Autodesk Inventor part; units mm, degrees
ref_plane "YZ Plane" through (0, 0, 0) normal (1, 0, 0) x (0, 1, 0)
ref_plane "XZ Plane" through (0, 0, 0) normal (0, 1, 0) x (-1, 0, 0)
ref_plane "XY Plane" through (0, 0, 0) normal (0, 0, 1) x (1, 0, 0)
sketch "Esboço1" plane through (0, 0, 0) normal (0, 0, 1) x (1, 0, 0)
  line L0 (0, 0) -> (40, 0)
  line L1 (40, 0) -> (40, 40)
  line L2 (40, 40) -> (0, 40)
  line L3 (0, 40) -> (0, 0)
  dimension "d0" = 40
  dimension "d1" = 40
extrude "Extrusão1" add sketch "Esboço1" along normal mid plane 5
sketch "Esboço2" plane through (0, 0, 2.5) normal (0, 0, 1) x (1, 0, 0)
  line L0 (0, 40) -> (0, 0)
  line L1 (0, 20) -> (40, 20)
  line L2 (40, 0) -> (40, 40)
  circle A0 centre (20, 20) radius 5
  dimension "d6" = 10
extrude "Extrusão2" add sketch "Esboço2" along normal blind 7.5
fillet "Arredondamento1" radius 1 1 edges at (15, 20, 10)
properties part number "base"
Could you check a few things on this model? Use its own coordinates, in mm. A direction names the side the tool comes from. Give positions to 0.01 mm unless a question says otherwise; leave off trailing zeros. Order: outer loops, then holes, each group sorted by start corner. A loop starts at its lowest first (then second) coordinate and runs counter-clockwise, first axis right, second up. Notation, with made-up numbers: (-39.75, -11.5) -> (-14.75, -11.5) arc R22 ccw to (-14.75, 24.5) -> close; hole circle Ø1 at (41.5, 39). An arc over 180 degrees is marked (long way). Answer in a Markdown table with one row per item. Add a question column.
Item 1: Imagine slicing it at D-D (y = 33.5). List the corners of the cut face in (x, z) for me, and give its area (3 significant figures).
Item 2: I'm going to push flat-ended pins straight in: P1, Ø1, axis at x = 34, y = 23.5, coming from the +Z side; P2, Ø12, axis at x = 11, y = 18.5, coming from the +Z side. Where does each tip first touch, or does it pass through?
Item 3: Please list where these lines run through material, in increasing order: probe 1 along Z at (x, y) = (20, 10.5); probe 2 along X at (y, z) = (16, 5); probe 3 along X at (y, z) = (19, 8.5).
Item 4: Imagine slicing it at C-C (z = 8.5). List the corners of the cut face in (x, y) for me, and give its area (3 significant figures).
Item 5: For faces 1 (the flat face through (40, 20, 0)), 2 (the cylindrical face through (18.92, 24.88, 5.7)), which set-ups out of +Z, -Z, +X, -X, +Y, -Y let a thin tool reach every point of the face, with its end or its side?
Item 6: Imagine slicing it at A-A (y = 20). List the corners of the cut face in (x, z) for me.
Result:
| question | item | result |
|---|---|---|
| 1 | outline | (0, -2.5) -> (40, -2.5) -> (40, 2.5) -> (0, 2.5) -> close |
| 1 | area | 200 mm2 |
| 2 | P1 | z = 2.5 |
| 2 | P2 | z = 10 |
| 3 | probe 1 | -2.5 to 2.5 |
| 3 | probe 2 | 17 to 23 |
| 3 | probe 3 | 15.1 to 24.9 |
| 4 | outline | circle Ø10 at (20, 20) |
| 4 | area | 78.5 mm2 |
| 5 | face 1 | +Z, -Z, +X, +Y, -Y |
| 5 | face 2 | +Z |
| 6 | outline | (0, -2.5) -> (40, -2.5) -> (40, 2.5) -> (25, 2.5) -> (25, 9) arc R1 ccw to (24, 10) -> (16, 10) arc R1 ccw to (15, 9) -> (15, 2.5) -> (0, 2.5) -> close |
